from build123d import *

# Parameters (mm, degrees)
F0_W        = 75
F0_H        = 30
F0_H_2      = 72.8525593877
F0_R        = 31.05
F1_DEPTH    = 30
F2_T1_DEPTH = 438.2716205132
F3_R        = 37.49999


# Not quite as in the source:
# - a fillet or chamfer that OpenCascade refuses, or shapes differently, is made with other operations: its cross-section is extruded or revolved along the edge and cut away or added
# - a fillet or chamfer is up to 0.001 mm smaller than in the source, because OpenCascade refuses the exact size


with BuildPart() as f1:
    # F0 (on Right) → F1 (new body, symmetric)
    with BuildSketch(Plane.YZ):
        with Locations((0, 51.4262796938)):
            Rectangle(F0_W, F0_H)
        Rectangle(F0_W, F0_H_2)
        Circle(F0_R, mode=Mode.SUBTRACT)
    extrude(amount=F1_DEPTH, both=True)

    # F2: chamfer of 70 x 24 on 2 edges, made by hand

    # F2_s2 → F2_t1 (cut)
    with BuildSketch(Plane.XZ.offset(-219.1358102566)):
        Polygon((30, 33.5737203062), (6, -36.4262796938), (30, -36.4262796938), align=None)
        Polygon((-6, -36.4262796938), (-30, 33.5737203062), (-30, -36.4262796938), align=None)
    extrude(amount=F2_T1_DEPTH, mode=Mode.SUBTRACT)

    # F3 (radius 37.5 in the source; OpenCascade refuses exactly that, so slightly less here)
    f3_edges = [f1.edges().sort_by_distance(p)[0] for p in [
        (0, -37.5, -36.42628),
        (0, 37.5, -36.42628),
    ]]
    fillet(f3_edges, radius=F3_R)


solid = f1.part
Can you work these out from the model? Positions are in its coordinate system, mm. Round coordinates to 2 decimals unless told otherwise and drop trailing zeros. Write each loop counter-clockwise with the first axis right and the second up, starting at its lowest first coordinate (ties: lowest second). Pieces come first, ordered by that corner, then holes. Notation, with made-up numbers: M 38,59.25 L 94,59.25 A11 cw 94,67.25 Z; hole C 27,-31.75 d11. An arc over 180 degrees is marked long. Use CSV: the item, a comma, the result in double quotes.
(1) Imagine slicing it at D-D (y = 23). Write out the boundary of the cut face in (x, z).
Check values:
outline,"M -30,33.57 L -25.64,20.86 L 25.64,20.86 L 30,33.57 L 30,66.43 L -30,66.43 Z; M -11.34,-20.86 L -8.7,-28.54 L 8.7,-28.54 L 11.34,-20.86 Z"
(2) I need wall thicknesses on line 1 along Y through (x, z) = (4, 0); line 2 along Z through (x, y) = (-9, 0); line 3 along Z through (x, y) = (1, 0). Which ranges of each line are inside material? Lowest first, please.
Check values:
line 1,"-37.48 to -31.05, 31.05 to 37.48"
line 2,"31.05 to 66.43"
line 3,"-36.43 to -31.05, 31.05 to 66.43"
(3) Imagine slicing it at C-C (x = 12.5). Write out the boundary of the cut face in (y, z), plus the area to 3 significant figures.
Check values:
outline,"M -37.5,1.07 A37.5 ccw -32.6,-17.47 L -25.67,-17.47 A31.05 cw long 25.67,-17.47 L 32.6,-17.47 A37.5 ccw 37.5,1.07 L 37.5,66.43 L -37.5,66.43 Z"
area,"3,690 mm^2"
(4) Imagine slicing it at A-A (y = 11). Write out the boundary of the cut face in (x, z), plus the area to 3 significant figures.
Check values:
outline,"M -30,33.57 L -28.44,29.04 L 28.44,29.04 L 30,33.57 L 30,66.43 L -30,66.43 Z; M -8.53,-29.04 L -6.57,-34.78 L 6.57,-34.78 L 8.53,-29.04 Z"
area,"2,320 mm^2"
(5) I'm going to push flat-ended pins straight in: pin 1 (1 mm diameter, centred on x = -22, y = -19.5, fed in from -Z); pin 2 (6 mm diameter, centred on x = 12, z = -19, fed in from +Y). Where does each tip first touch, or does it pass through?
Check values:
pin 1,"z = 23.75"
pin 2,"y = 33.39"
(6) Imagine slicing it at B-B (z = 13.5). Write out the boundary of the cut face in (x, y), plus the area to 3 significant figures.
Check values:
outline,"M -23.12,-37.5 L 23.12,-37.5 L 23.12,-27.96 L -23.12,-27.96 Z; M -23.12,27.96 L 23.12,27.96 L 23.12,37.5 L -23.12,37.5 Z"
area,"882 mm^2"
(7) We'd pull the mould along Z, two halves only. Please class faces 1 (the cylindrical face through (0.26, -30.95, -20.1)), 2 (the flat face through (0, -37.5, 34)), 3 (the cylindrical face through (-0.516, -4.042, 30.786)), 4 (the flat face through (0, -1, 66.426)): +Z half, -Z half, draft (parallel to the pull), parting line (faces both ways), or undercut.
Check values:
face 1,"-Z half"
face 2,"draft"
face 3,"undercut"
face 4,"+Z half"
